from build123d import *

# Parameters (mm, degrees)
SKETCH_1_W      = 290
SKETCH_1_H      = 195
EXTRUDE_1_DEPTH = 5
SKETCH_2_W      = 50
SKETCH_2_H      = 98
EXTRUDE_2_DEPTH = 5
FILLET_1_R      = 10
DRAFT_1_ANGLE   = 15
FILLET_2_R      = 2


with BuildPart() as part:
    # 草图1 → 凸台-拉伸1 (new body)
    with BuildSketch(Plane.XY):
        Rectangle(SKETCH_1_W, SKETCH_1_H)
    extrude(amount=EXTRUDE_1_DEPTH)

    # 草图2 → 凸台-拉伸2 (add)
    with BuildSketch(Plane.XY.offset(5)):
        with Locations((100, 11.5)):
            Rectangle(SKETCH_2_W, SKETCH_2_H)
    extrude(amount=EXTRUDE_2_DEPTH)

    # 圆角1
    fillet_1_edges = [part.edges().sort_by_distance(p)[0] for p in [
        (125, -37.5, 7.5),
        (125, 60.5, 7.5),
        (75, 60.5, 7.5),
        (75, -37.5, 7.5),
    ]]
    fillet(fillet_1_edges, radius=FILLET_1_R)

    # 拔模1
    draft_1_faces = [part.faces().sort_by_distance(p)[0] for p in [
        (75, 11.5, 7.5),
        (77.928932188, 57.571067812, 7.5),
        (100, 60.5, 7.5),
        (122.071067812, 57.571067812, 7.5),
        (125, 11.5, 7.5),
        (122.071067812, -34.571067812, 7.5),
        (100, -37.5, 7.5),
        (77.928932188, -34.571067812, 7.5),
    ]]
    draft(draft_1_faces, Plane.XY.offset(10), DRAFT_1_ANGLE)

    # 圆角2
    fillet_2_edges = [part.edges().sort_by_distance(p)[0] for p in [
        (100, 61.839745962, 5),
        (100, 60.5, 10),
        (126.339745962, 11.5, 5),
        (125, 11.5, 10),
        (75, 11.5, 10),
        (100, -37.5, 10),
        (77.928932188, -34.571067812, 10),
        (122.071067812, -34.571067812, 10),
        (77.928932188, 57.571067812, 10),
        (122.071067812, 57.571067812, 10),
        (73.660254038, 11.5, 5),
        (100, -38.839745962, 5),
        (123.018411267, 58.518411267, 5),
        (76.981588733, 58.518411267, 5),
        (123.018411267, -35.518411267, 5),
        (76.981588733, -35.518411267, 5),
    ]]
    fillet(fillet_2_edges, radius=FILLET_2_R)


solid = part.part
Here's how the part is built. I have some questions about the finished solid (model axes, mm). Give positions to 0.01 mm unless a question says otherwise; leave off trailing zeros. Write each loop counter-clockwise with the first axis right and the second up, starting at its lowest first coordinate (ties: lowest second). Pieces come first, ordered by that corner, then holes. Notation, with made-up numbers: (26, -19.75) -> (84, -19.75) arc R13 cw to (84, 3.25) -> close; hole circle Ø4 at (9.5, 27.25). An arc over 180 degrees is marked (long way). Use one line per item in the form item = value. Start each with the question number.
1. Will these pins go through, and if not, where does the flat tip stop? pin 1 Ø3 at (x, z) = (-105.5, 6) entering from -Y; pin 2 Ø2 at (x, y) = (62.5, 37) entering from +Z.
2. Imagine slicing it at C-C on y = -73. List the corners of the cut face in (x, z) for me.
3. Imagine slicing it at B-B on x = -27.5. List the corners of the cut face in (y, z) for me, plus the area to 3 significant figures.
4. Imagine slicing it at A-A on y = -1. List the corners of the cut face in (x, z) for me, plus the area to 3 significant figures.
5. If I drill on L1, parallel to Z at x = 17.5, y = -28.5; L2, parallel to X at y = 19, z = 9; L3, parallel to Z at x = 103, y = 59.5, over which ranges is the centre line in solid material (lowest first)?
Entries:
q1.pin_1 = -97.5
q1.pin_2 = 5
q2.outline = (-145, 0) -> (145, 0) -> (145, 5) -> (-145, 5) -> close
q3.outline = (-97.5, 0) -> (97.5, 0) -> (97.5, 5) -> (-97.5, 5) -> close
q3.area = 975 mm²
q4.outline = (-145, 0) -> (145, 0) -> (145, 5) -> (127.87, 5) arc R2 cw to (125.94, 6.48) -> (125.4, 8.52) arc R2 ccw to (123.47, 10) -> (76.53, 10) arc R2 ccw to (74.6, 8.52) -> (74.06, 6.48) arc R2 cw to (72.13, 5) -> (-145, 5) -> close
q4.area = 1,710 mm²
q5.L1 = 0 to 5
q5.L2 = 74.8 to 125.2
q5.L3 = 0 to 9.93
